Work out the finished part from the listing and answer in its coordinate system (mm). A direction names the side the tool comes from. Coordinates: 2 decimals unless noted, no trailing zeros. Write each loop counter-clockwise with the first axis right and the second up, starting at its lowest first coordinate (ties: lowest second). Pieces come first, ordered by that corner, then holes. Notation, with made-up numbers: (-16, -25) - (43, -25) arc R26 ccw to (43, -10) - close; hole circle Ø11 at (4.25, 73). An arc over 180 degrees is marked (long way). Use one line per item in the form item = value. Start each with the question number.
Item 1: Consider probe 1 along X at (y, z) = (0.5, 4.75); probe 2 along Z at (x, y) = (19, -2.5); probe 3 along Z at (x, y) = (37, 1). Determine where each line is inside the solid, lowest interval first.
Item 2: A cutting plane is placed at C-C (x = 32). Write down the section's boundary in (y, z).
Item 3: A cutting plane is placed at A-A (z = 0). Write down the section's boundary in (x, y), then the cut area to 3 significant figures.
Item 4: Given pin 1 (8 mm diameter, centred on x = 36.5, y = 2.5, fed in from -Z); pin 2 (6 mm diameter, centred on x = 26.5, z = 4.5, fed in from +Y); pin 3 (8 mm diameter, centred on x = 28, z = -2.5, fed in from +Y), each flat-ended and moving along its own axis, determine where each tip first touches the part or whether it passes through.
Item 5: For faces 1 (the flat face through (45, 0, 0)), 2 (the flat face through (2.1, -5, 0)), determine the directions among +Z, -Z, +X, -X, +Y, -Y from which every point of the face is accessible in a straight line to the end or side of a thin tool.
from build123d import *

# Parameters (mm, degrees)
FILLET1_R     = 0.5
CHAMFER1_SIZE = 0.8


with BuildPart() as part:
    # Sketch1 → Revolve1 (revolve)
    with BuildSketch(Plane.XY):
        Polygon((0, 0), (0, 6.8), (2.1, 6.8), (2.1, 4.7), (45, 4.7), (45, 0), align=None)
    revolve(axis=Axis((45, 0, 0), (-1, 0, 0)))

    # Fillet1
    fillet1_edges = [part.edges().sort_by_distance(p)[0] for p in [
        (2.1, -6.8, 0),
        (0, -6.8, 0),
    ]]
    fillet(fillet1_edges, radius=FILLET1_R)

    # Chamfer1
    chamfer1_edges = [part.edges().sort_by_distance(p)[0] for p in [
        (45, -4.7, 0),
    ]]
    chamfer(chamfer1_edges, length=CHAMFER1_SIZE)


solid = part.part
Answer:
q1.probe_1 = 0 to 2.1
q1.probe_2 = -3.98 to 3.98
q1.probe_3 = -4.59 to 4.59
q2.outline = circle Ø9.4 at (0, 0)
q3.outline = (0, -6.3) arc R0.5 ccw to (0.5, -6.8) - (1.6, -6.8) arc R0.5 ccw to (2.1, -6.3) - (2.1, -4.7) - (44.2, -4.7) - (45, -3.9) - (45, 3.9) - (44.2, 4.7) - (2.1, 4.7) - (2.1, 6.3) arc R0.5 ccw to (1.6, 6.8) - (0.5, 6.8) arc R0.5 ccw to (0, 6.3) - close
q3.area = 431 mm²
q4.pin_1 = -4.7
q4.pin_2 = 4.45
q4.pin_3 = 4.7
q5.face_1 = +Z, -Z, +X, +Y, -Y
q5.face_2 = +X
